Build history of the part. All positions in model axes, mm. Coordinates: 2 decimals unless noted, no trailing zeros. Write each loop counter-clockwise with the first axis right and the second up, starting at its lowest first coordinate (ties: lowest second). Pieces come first, ordered by that corner, then holes.
```python
from build123d import *

# Parameters (mm, degrees)
SKETCH1_W           = 37
SKETCH1_H           = 37
BOSS_EXTRUDE1_DEPTH = 546.5
SKETCH2_W           = 1.5
SKETCH2_H           = 20
SKETCH2_W_2         = 80
SKETCH2_H_2         = 2
SKETCH2_W_3         = 2
SKETCH2_H_3         = 6
CUT_EXTRUDE1_DEPTH  = 2.5
SKETCH3_W           = 20
SKETCH3_H           = 6
CUT_EXTRUDE2_DEPTH  = 1.5
SKETCH4_W           = 20
SKETCH4_H           = 2
CUT_EXTRUDE3_DEPTH  = 2
SKETCH5_R           = 3
CUT_EXTRUDE4_DEPTH  = 550.419921372
SKETCH6_R           = 3
CUT_EXTRUDE5_DEPTH  = 550.419921372
SKETCH7_R           = 10
CUT_EXTRUDE6_DEPTH  = 550.419921372
SKETCH8_W           = 18
SKETCH8_H           = 40
CUT_EXTRUDE7_DEPTH  = 10


with BuildPart() as part:
    # Sketch1 → Boss-Extrude1 (new body)
    with BuildSketch(Plane.XY):
        with BuildLine():
            Line((0.5, 0), (39.5, 0))
            ThreePointArc((39.5, 0), (39.853553391, 0.146446609), (40, 0.5))
            Line((40, 0.5), (40, 39.5))
            ThreePointArc((40, 39.5), (39.853553391, 39.853553391), (39.5, 40))
            Line((39.5, 40), (0.5, 40))
            ThreePointArc((0.5, 40), (0.146446609, 39.853553391), (0, 39.5))
            Line((0, 39.5), (0, 0.5))
            ThreePointArc((0, 0.5), (0.146446609, 0.146446609), (0.5, 0))
        make_face()
        with Locations((20, 20)):
            Rectangle(SKETCH1_W, SKETCH1_H, mode=Mode.SUBTRACT)
    extrude(amount=BOSS_EXTRUDE1_DEPTH)

    # Sketch2 → Cut-Extrude1 (cut)
    with BuildSketch(Plane.ZY):
        with Locations((0.75, 20)):
            Rectangle(SKETCH2_W, SKETCH2_H)
        with Locations((39.25, 20)):
            Rectangle(SKETCH2_W, SKETCH2_H)
        with Locations((507.25, 20)):
            Rectangle(SKETCH2_W, SKETCH2_H)
        with Locations((545.75, 20)):
            Rectangle(SKETCH2_W, SKETCH2_H)
        with Locations((446.5, 13)):
            Rectangle(SKETCH2_W_2, SKETCH2_H_2)
        with Locations((100, 13)):
            Rectangle(SKETCH2_W_2, SKETCH2_H_2)
        with Locations((154, 9)):
            Rectangle(SKETCH2_W_3, SKETCH2_H_3)
        with Locations((392.5, 9)):
            Rectangle(SKETCH2_W_3, SKETCH2_H_3)
        Polygon((40.1, 40), (26.243593539, 32), (6.143593539, 32), (20, 40), align=None)
        Polygon((520.256406461, 32), (540.356406461, 32), (526.5, 40), (506.4, 40), align=None)
    extrude(amount=-CUT_EXTRUDE1_DEPTH, mode=Mode.SUBTRACT)

    # Sketch3 → Cut-Extrude2 (cut)
    with BuildSketch(Plane(origin=(0, 40, 0), x_dir=(1, 0, 0), z_dir=(0, 1, 0))):
        with Locations((20, -469.5)):
            Rectangle(SKETCH3_W, SKETCH3_H)
        with Locations((20, -77)):
            Rectangle(SKETCH3_W, SKETCH3_H)
    extrude(amount=-CUT_EXTRUDE2_DEPTH, mode=Mode.SUBTRACT)

    # Sketch4 → Cut-Extrude3 (cut)
    with BuildSketch(Plane(origin=(0, 40, 0), x_dir=(1, 0, 0), z_dir=(0, 1, 0))):
        with Locations((20, -144.3)):
            Rectangle(SKETCH4_W, SKETCH4_H)
        with Locations((20, -182.3)):
            Rectangle(SKETCH4_W, SKETCH4_H)
        with Locations((20, -364.2)):
            Rectangle(SKETCH4_W, SKETCH4_H)
        with Locations((20, -402.2)):
            Rectangle(SKETCH4_W, SKETCH4_H)
    extrude(amount=-CUT_EXTRUDE3_DEPTH, mode=Mode.SUBTRACT)

    # Sketch5 → Cut-Extrude4 (cut, through all)
    with BuildSketch(Plane.XZ):
        with Locations(Location((10, 351.25, 0), (0, 0, 270))):
            Circle(SKETCH5_R)
        with Locations(Location((10, 195.25, 0), (0, 0, 270))):
            Circle(SKETCH5_R)
        with Locations(Location((10, 273.25, 0), (0, 0, 270))):
            Circle(SKETCH5_R)
    extrude(amount=-CUT_EXTRUDE4_DEPTH, mode=Mode.SUBTRACT)

    # Sketch6 → Cut-Extrude5 (cut, through all)
    with BuildSketch(Plane(origin=(0, 0, 0), x_dir=(-1, 0, 0), z_dir=(0, -1, 0))):
        with Locations(Location((-28, -436.5, 0), (0, 0, 90))):
            Circle(SKETCH6_R)
        with Locations(Location((-28, -326.5, 0), (0, 0, 90))):
            Circle(SKETCH6_R)
        with Locations(Location((-28, -220, 0), (0, 0, 90))):
            Circle(SKETCH6_R)
        with Locations(Location((-28, -110, 0), (0, 0, 90))):
            Circle(SKETCH6_R)
    extrude(amount=-CUT_EXTRUDE5_DEPTH, mode=Mode.SUBTRACT)

    # Sketch7 → Cut-Extrude6 (cut, through all)
    with BuildSketch(Plane.ZY):
        with Locations((273.25, 20)):
            Circle(SKETCH7_R)
    extrude(amount=-CUT_EXTRUDE6_DEPTH, mode=Mode.SUBTRACT)

    # Sketch8 → Cut-Extrude7 (cut)
    with BuildSketch(Plane(origin=(0, 40, 0), x_dir=(1, 0, 0), z_dir=(0, 1, 0))):
        with Locations((26, -273.25)):
            Rectangle(SKETCH8_W, SKETCH8_H)
    extrude(amount=-CUT_EXTRUDE7_DEPTH, mode=Mode.SUBTRACT)


solid = part.part
```
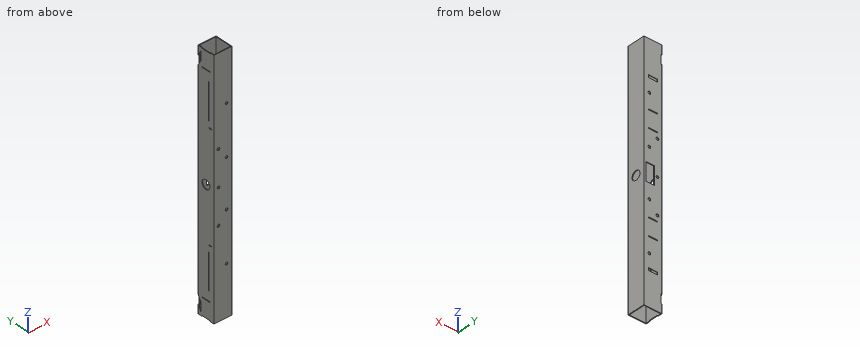
1. Saw through at B-B on y = 25. List the corners of the cut face in (x, z).
Computed values:
outline: (0, 1.5) - (1.5, 1.5) - (1.5, 38.5) - (0, 38.5) - close; (0, 40) - (1.5, 40) - (1.5, 264.59) - (0, 264.59) - close; (0, 281.91) - (1.5, 281.91) - (1.5, 506.5) - (0, 506.5) - close; (0, 508) - (1.5, 508) - (1.5, 545) - (0, 545) - close; (38.5, 0) - (40, 0) - (40, 264.59) - (38.5, 264.59) - close; (38.5, 281.91) - (40, 281.91) - (40, 546.5) - (38.5, 546.5) - close
2. Flat gauge pins, fed straight in: pin 1 (1.6 mm diameter, centred on x = 1, y = 20, fed in from +Z); pin 2 (1.6 mm diameter, centred on y = 39, z = 523, fed in from -X). Where does each tip first touch, or does it go through?
Computed values:
pin 1: stops at z = 545
pin 2: stops at x = 2.5
3. Saw through at A-A on z = 165. List the corners of the cut face in (x, y).
Computed values:
outline: (0, 0.5) arc R0.5 ccw to (0.5, 0) - (39.5, 0) arc R0.5 ccw to (40, 0.5) - (40, 39.5) arc R0.5 ccw to (39.5, 40) - (0.5, 40) arc R0.5 ccw to (0, 39.5) - close; hole (1.5, 1.5) - (38.5, 1.5) - (38.5, 38.5) - (1.5, 38.5) - close
4. Probe line 1 along Y through (x, z) = (29, 115); line 2 along X through (y, z) = (0.6, 195.25). List the from-to ranges inside material, lowest first.
Computed values:
line 1: y = 0 to 1.5, 38.5 to 40
line 2: x = 0 to 7, 13 to 40
